The model under review builds one solid part; all positions refer to its coordinate system, in mm. A direction names the side the tool comes from. Give positions to 0.01 mm unless a question says otherwise; leave off trailing zeros. Order: outer loops, then holes, each group sorted by start corner. A loop starts at its lowest first (then second) coordinate and runs counter-clockwise, first axis right, second up. Notation, with made-up numbers: M -24,-29.75 L 8,-29.75 A28 cw 8,7.25 Z; hole C 48.5,31.25 d10. An arc over 180 degrees is marked long. One line per question, with ' | ' between items. Start each with the question number.
1. We need section D-D on y = 12.5. Write out the cut boundary in (x, z).
2. Wall thickness on L1, parallel to Y at x = -12, z = 0.25; L2, parallel to Y at x = 14, z = 0.45; L3, parallel to X at y = -2.5, z = 1.25: over which ranges is each line inside the solid? List them lowest first.
3. We need section C-C on x = 1. Write out the cut boundary in (y, z), then the cut area to 3 significant figures.
4. The part is to be moulded in two halves that separate along X. For faces 1 (the face through (-9, -3.3, 1.5)), 2 (the face through (-11, -1.5, 1.5)), 3 (the face through (14.624, -14.644, 0.507)), 4 (the face through (-13, -3.3, 1.5)), say which applies: +X half, -X half, draft (parallel to the pull), parting line (faces both ways), or undercut.
5. We need section B-B on z = 1.6. Write out the cut boundary in (x, y).
6. Insertion check: P1, Ø0.8, axis at y = 11.5, z = 1.5, coming from the -X side; P2, Ø0.5, axis at y = 12, z = 1.5, coming from the +X side; P3, Ø0.5, axis at x = -2.5, z = 1.5, coming from the -Y side. Each pin has a flat end and moves straight along its axis. Give the tip position at first contact, or say it passes through.
7. For faces 5 (the face through (5, -0.1, 1.5)), 6 (the face through (6, 11, 1.5)), 7 (the face through (4, 12, 1.5)), 8 (the face through (6, 12, 2)), 9 (the face through (-0.1, -5, 1.5)), list the 3-axis set-ups (+Z, -Z, +X, -X, +Y, -Y) from which the entire face can be reached by the end or side of a thin tool; tool diameter is ignored.
8. We need section A-A on y = -2.54. Write out the cut boundary in (x, z).
```python
from build123d import *

# Parameters (mm, degrees)
SKETCH_1_W                 = 30
SKETCH_1_H                 = 30
EXTRUDE_1_DEPTH            = 1
FILLET_1_R                 = 1.25
SKETCH_2_R                 = 1.6
CUT_EXTRUDE_1_DEPTH        = 1
SKETCH_3_R                 = 0.5
CUT_EXTRUDE_2_DEPTH        = 1
PATTERN_LINEAR_1_COUNT     = 3
PATTERN_LINEAR_1_PITCH     = 2.54
PATTERN_LINEAR_1_COL_COUNT = 3
PATTERN_LINEAR_1_COL_PITCH = 2.54
SKETCH_4_W                 = 10
SKETCH_4_H                 = 10
EXTRUDE_2_DEPTH            = 1
SKETCH_5_W                 = 4
SKETCH_5_H                 = 3.5
SKETCH_5_H_2               = 2
EXTRUDE_3_DEPTH            = 1


with BuildPart() as part:
    # ｽｹｯﾁ1 → ﾎﾞｽ - 押し出し1 (new body)
    with BuildSketch(Plane.XY):
        Rectangle(SKETCH_1_W, SKETCH_1_H)
    extrude(amount=EXTRUDE_1_DEPTH)

    # ﾌｨﾚｯﾄ1
    fillet_1_edges = [part.edges().sort_by_distance(p)[0] for p in [
        (15, -15, 0.5),
        (-15, -15, 0.5),
        (-15, 15, 0.5),
        (15, 15, 0.5),
    ]]
    fillet(fillet_1_edges, radius=FILLET_1_R)

    # ｽｹｯﾁ2 → ｶｯﾄ - 押し出し1 (cut)
    with BuildSketch(Plane.XY.offset(1)):
        with Locations((-12, 12)):
            Circle(SKETCH_2_R)
        with Locations((12, 12)):
            Circle(SKETCH_2_R)
        with Locations((-12, -12)):
            Circle(SKETCH_2_R)
        with Locations((12, -12)):
            Circle(SKETCH_2_R)
    extrude(amount=-CUT_EXTRUDE_1_DEPTH, mode=Mode.SUBTRACT)

    # ｽｹｯﾁ3 → ｶｯﾄ - 押し出し2 (cut)
    with BuildSketch(Plane.XY.offset(1)):
        with Locations((14, 0)):
            Circle(SKETCH_3_R)
    cut_extrude_2 = extrude(amount=-CUT_EXTRUDE_2_DEPTH, mode=Mode.SUBTRACT)

    # 直線ﾊﾟﾀｰﾝ1: ｶｯﾄ - 押し出し2 ×3
    with Locations(*[(0, -i * PATTERN_LINEAR_1_PITCH, 0) for i in range(1, PATTERN_LINEAR_1_COUNT)]):
        add(cut_extrude_2, mode=Mode.SUBTRACT)

    # 直線ﾊﾟﾀｰﾝ1 col: ｶｯﾄ - 押し出し2 ×3
    with Locations(*[(0, i * PATTERN_LINEAR_1_COL_PITCH, 0) for i in range(1, PATTERN_LINEAR_1_COL_COUNT)]):
        add(cut_extrude_2, mode=Mode.SUBTRACT)

    # ｽｹｯﾁ4 → ﾎﾞｽ - 押し出し2 (add)
    with BuildSketch(Plane.XY.offset(1)):
        Rectangle(SKETCH_4_W, SKETCH_4_H)
    extrude(amount=EXTRUDE_2_DEPTH)

    # ｽｹｯﾁ5 → ﾎﾞｽ - 押し出し3 (add)
    with BuildSketch(Plane.XY.offset(1)):
        with Locations((-11, -3.25)):
            Rectangle(SKETCH_5_W, SKETCH_5_H)
        with Locations((6, 12)):
            Rectangle(SKETCH_5_W, SKETCH_5_H_2)
    extrude(amount=EXTRUDE_3_DEPTH)


solid = part.part
```
Entries:
1) outline: M -15,0 L -13.52,0 L -13.52,1 L -15,1 Z; M -10.48,0 L 10.48,0 L 10.48,1 L 8,1 L 8,2 L 4,2 L 4,1 L -10.48,1 Z; M 13.52,0 L 15,0 L 15,1 L 13.52,1 Z
2) L1: y = -15 to -13.6, -10.4 to 10.4, 13.6 to 15 | L2: y = -14.97 to -5.58, -4.58 to -3.04, -2.04 to -0.5, 0.5 to 2.04, 3.04 to 4.58, 5.58 to 14.97 | L3: x = -13 to -9, -5 to 5
3) outline: M -15,0 L 15,0 L 15,1 L 5,1 L 5,2 L -5,2 L -5,1 L -15,1 Z | area: 40.0 mm^2
4) face 1: undercut | face 2: draft | face 3: +X half | face 4: -X half
5) outline: M -13,-5 L -9,-5 L -9,-1.5 L -13,-1.5 Z; M -5,-5 L 5,-5 L 5,5 L -5,5 Z; M 4,11 L 8,11 L 8,13 L 4,13 Z
6) P1: stops at x = 4 | P2: stops at x = 8 | P3: stops at y = -5
7) face 5: +Z, +X, -Y | face 6: +Z, +X, -X | face 7: +Z, -X, +Y | face 8: +Z, +X, -X, +Y, -Y | face 9: +Z, +X, -X, -Y
8) outline: M -15,0 L 13.5,0 L 13.5,1 L 5,1 L 5,2 L -5,2 L -5,1 L -9,1 L -9,2 L -13,2 L -13,1 L -15,1 Z; M 14.5,0 L 15,0 L 15,1 L 14.5,1 Z
